```python
from build123d import *

# Parameters (mm, degrees)
BOSS_EXTRUDE1_DEPTH = 3.8


with BuildPart() as part:
    # Sketch1 → Boss-Extrude1 (new body)
    with BuildSketch(Plane.XY):
        Polygon((0, 0), (7.6, 0), (7.6, 4), (10.6, 4), (10.6, 8), (7.6, 8), (7.6, 12), (0, 12), (0, 8), (-3, 8), (-3, 4), (0, 4), align=None)
        Polygon((7, 6), (5.5, 8.598076211), (2.5, 8.598076211), (1, 6), (2.5, 3.401923789), (5.5, 3.401923789), align=None, mode=Mode.SUBTRACT)
    extrude(amount=BOSS_EXTRUDE1_DEPTH)


solid = part.part
```
Part model, mm, in its own coordinate system. A direction names the side the tool comes from. Round coordinates to 2 decimals unless told otherwise and drop trailing zeros. Loops run counter-clockwise (first coordinate to the right, second up) from the corner with the lowest first, then second, coordinate; pieces in that order, holes last. Notation, with made-up numbers: (17, 78.25) -> (25, 78.25) arc R20 cw to (25, 111.25) -> close; hole circle Ø3 at (45.25, 25). An arc over 180 degrees is marked (long way). Use a Markdown table: item, result.
1) Tool access for faces 4 (the flat face through (4, 8.598, 2)), 5 (the flat face through (9, 4, 2)), 6 (the flat face through (-1, 8, 2)): list every direction of +Z, -Z, +X, -X, +Y, -Y with a clear straight run to the whole face (end or side of a thin tool).
The answers:
| item | result |
|---|---|
| face 4 | +Z, -Z |
| face 5 | +Z, -Z, +X, -Y |
| face 6 | +Z, -Z, -X, +Y |
2) Cut at A-A, the plane x = 1.75. List the corners of the cut face in (y, z).
The answers:
| item | result |
|---|---|
| outline | (0, 0) -> (4.7, 0) -> (4.7, 3.8) -> (0, 3.8) -> close; (7.3, 0) -> (12, 0) -> (12, 3.8) -> (7.3, 3.8) -> close |
3) Cut at B-B, the plane z = 2.55. List the corners of the cut face in (x, y), and give its area (3 significant figures).
The answers:
| item | result |
|---|---|
| outline | (-3, 4) -> (0, 4) -> (0, 0) -> (7.6, 0) -> (7.6, 4) -> (10.6, 4) -> (10.6, 8) -> (7.6, 8) -> (7.6, 12) -> (0, 12) -> (0, 8) -> (-3, 8) -> close; hole (1, 6) -> (2.5, 3.4) -> (5.5, 3.4) -> (7, 6) -> (5.5, 8.6) -> (2.5, 8.6) -> close |
| area | 91.8 mm2 |
4) Cut at D-D, the plane x = -0.5. List the corners of the cut face in (y, z), and give its area (3 significant figures).
The answers:
| item | result |
|---|---|
| outline | (4, 0) -> (8, 0) -> (8, 3.8) -> (4, 3.8) -> close |
| area | 15.2 mm2 |
5) Pull direction X, two halves, no side cores. Call faces 1 (the flat face through (1.76, 7.32, 1.87)), 2 (the flat face through (4, 9, 3.8)), 3 (the flat face through (-3, 6, 2)): pulls with the +X half, pulls with the -X half, needs draft (parallel to the pull), parting line crosses it, or undercut.
The answers:
| item | result |
|---|---|
| face 1 | undercut |
| face 2 | needs draft |
| face 3 | pulls with the -X half |
6) Cut at C-C, the plane y = 7. List the corners of the cut face in (x, z).
The answers:
| item | result |
|---|---|
| outline | (-3, 0) -> (1.58, 0) -> (1.58, 3.8) -> (-3, 3.8) -> close; (6.42, 0) -> (10.6, 0) -> (10.6, 3.8) -> (6.42, 3.8) -> close |
7) Drop flat-ended pins along their axis: pin 1 Ø1.1 at (y, z) = (9.5, 2) entering from -X; pin 2 Ø1.5 at (y, z) = (3, 1.5) entering from +X; pin 3 Ø1.5 at (x, z) = (8.5, 1) entering from -Y. Give the stop position or say it passes through.
The answers:
| item | result |
|---|---|
| pin 1 | stops at x = 0 |
| pin 2 | stops at x = 7.6 |
| pin 3 | stops at y = 4 |
8) Probe line 1 (X direction, y = 2.5, z = 1.8); line 2 (Y direction, x = 3.25, z = 2.8); line 3 (X direction, y = 7.5, z = 0.2). List the from-to ranges inside material, lowest first. Write a range as [from, to].
The answers:
| item | result |
|---|---|
| line 1 | x = [0, 7.6] |
| line 2 | y = [0, 3.4], [8.6, 12] |
| line 3 | x = [-3, 1.87], [6.13, 10.6] |
